Build history of the part. All positions in model axes, mm. A direction names the side the tool comes from. Round coordinates to 2 decimals unless told otherwise and drop trailing zeros. Order: outer loops, then holes, each group sorted by start corner. A loop starts at its lowest first (then second) coordinate and runs counter-clockwise, first axis right, second up. Notation, with made-up numbers: M 16,18 L 68,18 A25 ccw 68,57 Z; hole C 88.5,62 d1. An arc over 180 degrees is marked long. One line per question, with ' | ' between items. Start each with the question number.
from build123d import *

# Parameters (mm, degrees)
F0_W     = 30
F0_H     = 3
F0_W_2   = 3
F0_H_2   = 4.7552157193
F0_H_3   = 7
F1_DEPTH = 15
F2_R     = 2
F3_SIZE  = 5
F4_R     = 2
F5_R     = 3
F6_R     = 2.99999
F7_R     = 2.99999
F8_R     = 2
F9_R     = 2


# Not quite as in the source:
# - a fillet or chamfer is up to 0.001 mm smaller than in the source, because OpenCascade refuses the exact size


with BuildPart() as f1:
    # F0 (on Top) → F1 (new body)
    with BuildSketch(Plane.XY):
        with Locations((-15, -1.5)):
            Rectangle(F0_W, F0_H)
        Polygon((3, 0), (0, 0), (0, -3), (0, -33), (3, -33), (3, -3), align=None)
        Polygon((10, 0), (3, 0), (3, -3), (43, -3), (43, 0), (40, 0), (13, 0), align=None)
        with Locations((11.5, 2.3776078597)):
            Rectangle(F0_W_2, F0_H_2)
        with Locations((41.5, 3.5)):
            Rectangle(F0_W_2, F0_H_3)
    extrude(amount=F1_DEPTH)

    # F2
    f2_edges = [f1.edges().sort_by_distance(p)[0] for p in [
        (0, -3, 7.5),
    ]]
    fillet(f2_edges, radius=F2_R)

    # F3
    f3_edges = [f1.edges().sort_by_distance(p)[0] for p in [
        (3, -3, 7.5),
    ]]
    chamfer(f3_edges, length=F3_SIZE)

    # F4
    f4_edges = [f1.edges().sort_by_distance(p)[0] for p in [
        (13, 0, 7.5),
        (40, 0, 7.5),
        (10, 0, 7.5),
    ]]
    fillet(f4_edges, radius=F4_R)

    # F5
    f5_edges = [f1.edges().sort_by_distance(p)[0] for p in [
        (43, -3, 7.5),
    ]]
    fillet(f5_edges, radius=F5_R)

    # F6 (radius 3 in the source; OpenCascade refuses exactly that, so slightly less here)
    f6_edges = [f1.edges().sort_by_distance(p)[0] for p in [
        (-30, 0, 7.5),
    ]]
    fillet(f6_edges, radius=F6_R)

    # F7 (radius 3 in the source; OpenCascade refuses exactly that, so slightly less here)
    f7_edges = [f1.edges().sort_by_distance(p)[0] for p in [
        (3, -33, 7.5),
    ]]
    fillet(f7_edges, radius=F7_R)

    # F8
    f8_edges = [f1.edges().sort_by_distance(p)[0] for p in [
        (8, -3, 7.5),
    ]]
    fillet(f8_edges, radius=F8_R)

    # F9
    f9_edges = [f1.edges().sort_by_distance(p)[0] for p in [
        (3, -8, 7.5),
    ]]
    fillet(f9_edges, radius=F9_R)


solid = f1.part
Item 1: Flat gauge pins, fed straight in: pin 1 (2 mm diameter, centred on y = -16, z = 10, fed in from +X); pin 2 (3 mm diameter, centred on x = -10, z = 13, fed in from -Y); pin 3 (7.5 mm diameter, centred on x = 25, z = 4.5, fed in from +Y). Where does each tip first touch, or does it go through?
Item 2: Two-plate mould, pull along X, no slides. Class faces 4 (the face through (40, 4, 7)), 5 (the face through (3, -20, 7)), 6 (the face through (41, 7, 7)), 7 (the face through (13.6, 0.57, 7.6)): +X half, -X half, draft (parallel to the pull), parting line (faces both ways), or undercut.
Item 3: Cut at B-B on x = 11. Write the cut outline in (y, z), then the cut area to 3 significant figures.
Item 4: Cut at C-C on y = -20. Write the cut outline in (x, z).
Item 5: Tool access for faces 1 (the face through (13, 3, 7)), 2 (the face through (-9, 0, 7)), 3 (the face through (0, -19, 7)): list every direction of +Z, -Z, +X, -X, +Y, -Y with a clear straight run to the whole face (end or side of a thin tool).
Item 6: Wall check: line 1 along X through (y, z) = (-21.5, 2); line 2 along Y through (x, z) = (16.5, 6.5); line 3 along X through (y, z) = (5.5, 7). Give the ranges that are in metal, low to high. Write a range as [from, to].
Results found:
1) pin 1: stops at x = 3 | pin 2: stops at y = -3 | pin 3: stops at y = 0
2) face 4: undercut | face 5: +X half | face 6: draft | face 7: undercut
3) outline: M -3,0 L 4.76,0 L 4.76,15 L -3,15 Z | area: 116 mm^2
4) outline: M 0,0 L 3,0 L 3,15 L 0,15 Z
5) face 1: +Z, -Z, +Y | face 2: +Z, -Z, -X, +Y | face 3: +Z, -Z, -X, -Y
6) line 1: x = [0, 3] | line 2: y = [-3, 0] | line 3: x = [40, 43]
